Drawing for the job (mm, zero at the part's lowest x, y, z). Round coordinates to 2 decimals unless told otherwise and drop trailing zeros. Write each loop counter-clockwise with the first axis right and the second up, starting at its lowest first coordinate (ties: lowest second). Pieces come first, ordered by that corner, then holes. Notation, with made-up numbers: (76.25, 61.25) - (86.25, 61.25) arc R16 ccw to (86.25, 89.25) - close; hole circle Ø9 at (69.25, -15.5). An arc over 180 degrees is marked (long way). One line per question, with ' | ' between items.
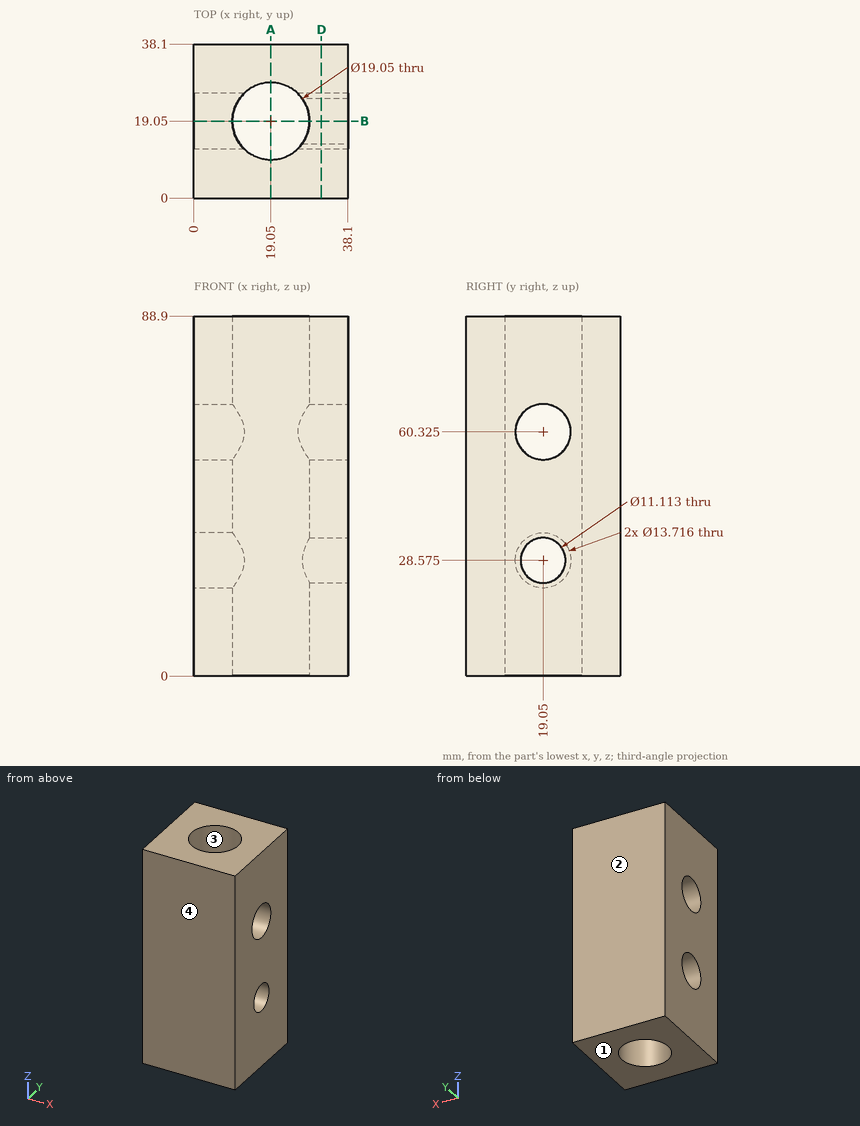
Q1. Pull direction Y, two halves, no side cores. Call the marked faces 1, 2, 3 and 4: +Y half, -Y half, draft (parallel to the pull), parting line (faces both ways), or undercut.
Found:
face 1: draft | face 2: +Y half | face 3: undercut | face 4: -Y half
Q2. Drop a flat-ended pin along its axis: pin 1 (5 mm diameter, centred on y = 16, z = 30.5, fed in from -X). Give the stop position or say it passes through.
Found:
pin 1: x = 26.79
Q3. Drill centre lines: L1, parallel to Z at x = 4.75, y = 19.05; L2, parallel to Z at x = 35, y = 19.05; L3, parallel to Y at x = 29, z = 29. Where is each one in solid material? Low to high. Write a range as from..to.
Found:
L1: 0..21.72, 35.43..53.47, 67.18..88.9 | L2: 0..23.02, 34.13..53.47, 67.18..88.9 | L3: 0..13.51, 24.59..38.1
Q4. Saw through at B-B, the plane y = 19.05. List the corners of the cut face in (x, z) (1 decimal), then the cut area to 3 significant figures.
Found:
outline: (0, 0) - (9.5, 0) - (9.5, 21.7) - (0, 21.7) - close; (0, 35.4) - (9.5, 35.4) - (9.5, 53.5) - (0, 53.5) - close; (0, 67.2) - (9.5, 67.2) - (9.5, 88.9) - (0, 88.9) - close; (28.6, 0) - (38.1, 0) - (38.1, 23) - (28.6, 23) - close; (28.6, 34.1) - (38.1, 34.1) - (38.1, 53.5) - (28.6, 53.5) - close; (28.6, 67.2) - (38.1, 67.2) - (38.1, 88.9) - (28.6, 88.9) - close | area: 1,200 mm^2
Q5. Saw through at D-D, the plane x = 31.5. State how many separate pieces and enclosed holes the cut face has, then the cut area to 3 significant figures.
Found:
separate pieces: 1 | enclosed holes: 2 | area: 3,140 mm^2
Q6. Saw through at A-A, the plane x = 19.05. List the corners of the cut face in (y, z) (1 decimal).
Found:
outline: (0, 0) - (9.5, 0) - (9.5, 88.9) - (0, 88.9) - close; (28.6, 0) - (38.1, 0) - (38.1, 88.9) - (28.6, 88.9) - close
